Could you check a few things on this model? Use its own coordinates, in mm. A direction names the side the tool comes from. Coordinates: 2 decimals unless noted, no trailing zeros. Loops run counter-clockwise (first coordinate to the right, second up) from the corner with the lowest first, then second, coordinate; pieces in that order, holes last. Notation, with made-up numbers: M -21.5,32 L 1.5,32 A22 cw 1.5,71 Z; hole C -11.75,-24 d2. An arc over 180 degrees is marked long. Write each question's results on one line, items separated by ' | '.
```python
from build123d import *

# Parameters (mm, degrees)
F0_W          = 101.6
F0_H          = 863.6
F1_DEPTH      = 4.7625
F2_R          = 8.25
F3_DEPTH      = 9.526
F5_DEPTH      = 9.526
F6_R          = 16
F8_DEPTH      = 4.7635
F8_DEPTH_BACK = 4.7635
F10_D         = 16.75


with BuildPart() as f1:
    # F0 (on Right) → F1 (new body, symmetric)
    with BuildSketch(Plane.YZ):
        with Locations((50.8, 431.8)):
            Rectangle(F0_W, F0_H)
    extrude(amount=F1_DEPTH, both=True)

    # F2 (on face) → F3 (cut, through all)
    with BuildSketch(Plane(origin=(-4.7625, 0, 0), x_dir=(0, -1, 0), z_dir=(-1, 0, 0))):
        with Locations((-50.8, 45)):
            Circle(F2_R)
        with Locations((-50.8, 440)):
            Circle(F2_R)
    extrude(amount=-F3_DEPTH, mode=Mode.SUBTRACT)

    # F4 (on face) → F5 (cut, through all)
    with BuildSketch(Plane.YZ.offset(4.7625)):
        Polygon((59, 821.8375473243), (0, 798), (0, 744.0732628661), (59, 767.9108101904), align=None)
    extrude(amount=-F5_DEPTH, mode=Mode.SUBTRACT)

    # F6
    f6_edges = [f1.edges().sort_by_distance(p)[0] for p in [
        (0, 59, 767.91081),
        (0, 59, 821.837547),
    ]]
    fillet(f6_edges, radius=F6_R)

    # F7 (on Right) → F8 (cut, two sides)
    with BuildSketch(Plane.YZ) as f8_sk:
        Polygon((0, 22.540836587), (0, 0), (55.4036807783, 0), (24, 7.250110976), (24, 17), align=None)
    extrude(amount=-F8_DEPTH, mode=Mode.SUBTRACT)
    extrude(f8_sk.sketch, amount=F8_DEPTH_BACK, mode=Mode.SUBTRACT)

    # F10 (through all)
    with Locations(Plane.YZ.offset(4.7625)):
        with Locations((50.8, 731), (50.8, 661), (13.2422749771, 660.3641925713)):
            Hole(F10_D / 2)


solid = f1.part
```
(1) Please list where these lines run through material, in increasing order: probe 1 along Y at (x, z) = (2.5, 661) (3 decimals); probe 2 along Z at (x, y) = (-1.25, 48.5); probe 3 along Z at (x, y) = (-1, 55). Write a range as from..to.
Reported:
probe 1: y = 0..4.891, 21.593..42.425, 59.175..101.6 | probe 2: z = 1.59..37.08, 52.92..432.08, 447.92..652.95, 669.05..722.95, 739.05..763.67, 813.14..863.6 | probe 3: z = 0.09..37.9, 52.1..432.9, 447.1..653.75, 668.25..723.75, 738.25..768.12, 808.7..863.6
(2) If we mould it in two halves opening along Z, with no side actions, what happens to faces 4 (the cylindrical face through (-0.07, 15.06, 652.19)), 5 (the flat face through (-4.762, 61, 438))? For each: released by +Z, released by -Z, zero draft, split by the parting line, or undercut.
Reported:
face 4: undercut | face 5: zero draft
(3) Imagine slicing it at C-C, the plane z = 731. List the corners of the cut face in (x, y) for me (1 decimal), and give its area (3 significant figures).
Reported:
outline: M -4.8,0 L 4.8,0 L 4.8,42.4 L -4.8,42.4 Z; M -4.8,59.2 L 4.8,59.2 L 4.8,101.6 L -4.8,101.6 Z | area: 808 mm2
(4) Will these pins go through, and if not, where does the flat tip stop? P1, Ø5, axis at x = 0, z = 10.5, coming from the -Y side; P2, Ø5, axis at x = 2, z = 793, coming from the -Y side.
Reported:
P1: stops at y = 24 | P2: stops at y = 59
(5) Imagine slicing it at B-B, the plane x = 2.25. List the corners of the cut face in (y, z) for me (3 decimals).
Reported:
outline: M 0,22.541 L 24,17 L 24,7.25 L 55.404,0 L 101.6,0 L 101.6,863.6 L 0,863.6 L 0,798 L 37.006,812.952 A16 cw 59,798.117 L 59,778.703 A16 cw 48.994,763.868 L 0,744.073 Z; hole C 13.242,660.364 d16.75; hole C 50.8,661 d16.75; hole C 50.8,731 d16.75; hole C 50.8,45 d16.5; hole C 50.8,440 d16.5
(6) Imagine slicing it at A-A, the plane z = 45. List the corners of the cut face in (x, y) for me, and give its area (3 significant figures).
Reported:
outline: M -4.76,0 L 4.76,0 L 4.76,42.55 L -4.76,42.55 Z; M -4.76,59.05 L 4.76,59.05 L 4.76,101.6 L -4.76,101.6 Z | area: 811 mm2
(7) Which directions (+Z, -Z, +X, -X, +Y, -Y) give clear straight access to the entire face, cutting with the end or side of a thin tool? Please do faces 1 (the flat face through (0.07, 18.76, 805.58)), 2 (the flat face through (0.07, 24.15, 753.83)), 3 (the flat face through (4.762, 61, 438)).
Reported:
face 1: +X, -X | face 2: +X, -X, -Y | face 3: +Z, -Z, +X, +Y, -Y
